```python
from build123d import *

# Parameters (mm, degrees)
CROQUIS1_W              = 47
CROQUIS1_H              = 47
CROQUIS1_R              = 1.65
SALIENTE_EXTRUIR1_DEPTH = 5.5
CORTAR_EXTRUIR1_DEPTH   = 2.35
CROQUIS7_R              = 12.35
CORTAR_EXTRUIR2_DEPTH   = 5.5
CROQUIS8_R              = 1.7
CORTAR_EXTRUIR3_DEPTH   = 5.5
CROQUIS9_R              = 3.25
CORTAR_EXTRUIR4_DEPTH   = 2.5
REDONDEO1_R             = 10


with BuildPart() as part:
    # Croquis1 → Saliente-Extruir1 (new body)
    with BuildSketch(Plane(origin=(0, 0, 0), x_dir=(0, 0, -1), z_dir=(1, 0, 0))):
        Rectangle(CROQUIS1_W, CROQUIS1_H)
        with Locations((-15.5, 15.5)):
            Circle(CROQUIS1_R, mode=Mode.SUBTRACT)
        with Locations((15.5, 15.5)):
            Circle(CROQUIS1_R, mode=Mode.SUBTRACT)
        with Locations((15.5, -15.5)):
            Circle(CROQUIS1_R, mode=Mode.SUBTRACT)
        with Locations((-15.5, -15.5)):
            Circle(CROQUIS1_R, mode=Mode.SUBTRACT)
    extrude(amount=SALIENTE_EXTRUIR1_DEPTH)

    # Croquis2 → Cortar-Extruir1 (cut)
    with BuildSketch(Plane(origin=(5.5, 0, 0), x_dir=(0, 0, -1), z_dir=(1, 0, 0))):
        Polygon((0, 13.968911087), (2.625, 15.484455543), (2.625, 18.515544457), (0, 20.031088913), (-2.625, 18.515544457), (-2.625, 15.484455543), align=None)
        Polygon((14.722431864, -11.531088913), (17.347431864, -10.015544457), (17.347431864, -6.984455543), (14.722431864, -5.468911087), (12.097431864, -6.984455543), (12.097431864, -10.015544457), align=None)
        Polygon((-17.347431864, -6.984455543), (-17.347431864, -10.015544457), (-14.722431864, -11.531088913), (-12.097431864, -10.015544457), (-12.097431864, -6.984455543), (-14.722431864, -5.468911087), align=None)
    extrude(amount=-CORTAR_EXTRUIR1_DEPTH, mode=Mode.SUBTRACT)

    # Croquis7 → Cortar-Extruir2 (cut)
    with BuildSketch(Plane(origin=(5.5, 0, 0), x_dir=(0, 0, -1), z_dir=(1, 0, 0))):
        Circle(CROQUIS7_R)
    extrude(amount=-CORTAR_EXTRUIR2_DEPTH, mode=Mode.SUBTRACT)

    # Croquis8 → Cortar-Extruir3 (cut)
    with BuildSketch(Plane(origin=(5.5, 0, 0), x_dir=(0, 0, -1), z_dir=(1, 0, 0))):
        with Locations((0, 17)):
            Circle(CROQUIS8_R)
        with Locations((14.722431864, -8.5)):
            Circle(CROQUIS8_R)
        with Locations((-14.722431864, -8.5)):
            Circle(CROQUIS8_R)
    extrude(amount=-CORTAR_EXTRUIR3_DEPTH, mode=Mode.SUBTRACT)

    # Croquis9 → Cortar-Extruir4 (cut)
    with BuildSketch(Plane.ZY):
        with Locations((-15.5, -15.5)):
            Circle(CROQUIS9_R)
        with Locations((-15.5, 15.5)):
            Circle(CROQUIS9_R)
        with Locations((15.5, 15.5)):
            Circle(CROQUIS9_R)
        with Locations((15.5, -15.5)):
            Circle(CROQUIS9_R)
    extrude(amount=-CORTAR_EXTRUIR4_DEPTH, mode=Mode.SUBTRACT)

    # Redondeo1
    redondeo1_edges = [part.edges().sort_by_distance(p)[0] for p in [
        (2.75, -23.5, 23.5),
        (2.75, 23.5, 23.5),
        (2.75, 23.5, -23.5),
        (2.75, -23.5, -23.5),
    ]]
    fillet(redondeo1_edges, radius=REDONDEO1_R)


solid = part.part
```
Model file for the job. Use its own axes, mm. A direction names the side the tool comes from. Round coordinates to 2 decimals unless told otherwise and drop trailing zeros. Write each loop counter-clockwise with the first axis right and the second up, starting at its lowest first coordinate (ties: lowest second). Pieces come first, ordered by that corner, then holes. Notation, with made-up numbers: (73, 72) - (90, 72) arc R21 cw to (90, 99) - close; hole circle Ø8 at (76, -24). An arc over 180 degrees is marked (long way). One line per item, written item: value.
(1) 3-axis set-ups, long thin cutter, end or side, ignore diameter. For faces 5 (the flat face through (2.5, 14, -14)), 6 (the flat face through (4.34, -6.22, 16.02)), 7 (the cylindrical face through (3.979, -15.004, 13.926)): which of +Z, -Z, +X, -X, +Y, -Y reach the whole face in a straight line?
Values follow:
face 5: -X
face 6: +X
face 7: +X, -X
(2) Two-plate mould, pull along Y, no slides. Class faces 1 (the flat face through (4, 17, 2.625)), 2 (the flat face through (3, 0, 23.5)), 3 (the cylindrical face through (2.79, -20.65, -20.49)), 4 (the cylindrical face through (1.232, -12.278, -15.923)): pulls with the +Y half, pulls with the -Y half, needs draft (parallel to the pull), parting line crosses it, or undercut.
Values follow:
face 1: undercut
face 2: needs draft
face 3: pulls with the -Y half
face 4: undercut
(3) Cut at C-C, the plane z = 15.5. Give the cut face in (x, y), plus the area to 3 significant figures.
Values follow:
outline: (0, -23.3) - (5.5, -23.3) - (5.5, -17.15) - (2.5, -17.15) - (2.5, -18.75) - (0, -18.75) - close; (0, -12.25) - (2.5, -12.25) - (2.5, -13.85) - (5.5, -13.85) - (5.5, -11.08) - (3.15, -11.08) - (3.15, -10.01) - (0, -10.01) - close; (0, -6.99) - (3.15, -6.99) - (3.15, -5.92) - (5.5, -5.92) - (5.5, 13.85) - (2.5, 13.85) - (2.5, 12.25) - (0, 12.25) - close; (0, 18.75) - (2.5, 18.75) - (2.5, 17.15) - (5.5, 17.15) - (5.5, 23.3) - (0, 23.3) - close
area: 182 mm²
(4) Drop flat-ended pins along their axis: P1, Ø2, axis at y = -16.5, z = 16, coming from the -X side; P2, Ø1.9, axis at x = 5, y = 17, coming from the -Z side; P3, Ø2.5, axis at y = -8.5, z = -14, coming from the +X side. Give the stop position or say it passes through.
Values follow:
P1: stops at x = 2.5
P2: stops at z = -23.17
P3: stops at x = 3.15
(5) Wall check: probe 1 along Y at (x, z) = (0.65, -15.5); probe 2 along Y at (x, z) = (3.35, 15.5); probe 3 along Z at (x, y) = (0.2, -9.5). Give the ranges that are in metal, low to high.
Values follow:
probe 1: y = -23.3 to -18.75, -12.25 to -10.01, -6.99 to 12.25, 18.75 to 23.3
probe 2: y = -23.3 to -17.15, -13.85 to -11.08, -5.92 to 13.85, 17.15 to 23.3
probe 3: z = -23.5 to -16.1, -13.35 to -7.89, 7.89 to 13.35, 16.1 to 23.5
(6) Cut at A-A, the plane x = 4.1. Give the number of separate pieces and of enclosed holes in the cut face, plus the area to 3 significant figures.
Values follow:
separate pieces: 1
enclosed holes: 8
area: 1,540 mm²
(7) Cut at D-D, the plane z = 21.5. Give the cut face in (x, y).
Values follow:
outline: (0, -19.5) - (5.5, -19.5) - (5.5, 19.5) - (0, 19.5) - close
(8) Cut at B-B, the plane y = 0. Give the cut face in (x, z), plus the area to 3 significant figures.
Values follow:
outline: (0, -23.5) - (5.5, -23.5) - (5.5, -12.35) - (0, -12.35) - close; (0, 12.35) - (5.5, 12.35) - (5.5, 23.5) - (0, 23.5) - close
area: 123 mm²
